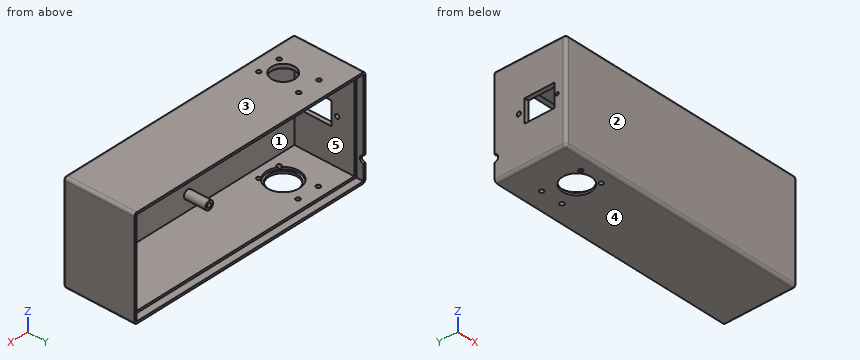
from build123d import *

# Parameters (mm, degrees)
SKETCH1_W           = 176
SKETCH1_H           = 70
BOSS_EXTRUDE1_DEPTH = 50
SKETCH2_W           = 170
SKETCH2_H           = 64
CUT_EXTRUDE1_DEPTH  = 47
SKETCH3_W           = 173
SKETCH3_H           = 67
CUT_EXTRUDE2_DEPTH  = 5
SKETCH4_R           = 3
SKETCH4_R_2         = 1.5
BOSS_EXTRUDE2_DEPTH = 15
CUT_EXTRUDE3_REACH  = 72
SKETCH5_R           = 10
SKETCH5_R_2         = 1.5
SKETCH6_R           = 11.5
CUT_EXTRUDE4_DEPTH  = 1.5
CUT_EXTRUDE5_REACH  = 72
SKETCH7_R           = 8.25
SKETCH7_R_2         = 1.5
SKETCH8_R           = 8.5
CUT_EXTRUDE6_DEPTH  = 1
FILLET1_R           = 2
CUT_EXTRUDE7_REACH  = 178
SKETCH9_R           = 1.5
SKETCH9_R_2         = 1
SKETCH9_W           = 16
SKETCH9_H           = 21
CUT_EXTRUDE8_REACH  = 178
SKETCH10_R          = 2.5


with BuildPart() as part:
    # Sketch1 → Boss-Extrude1 (new body)
    with BuildSketch(Plane(origin=(0, 0, 0), x_dir=(1, 0, 0), z_dir=(0, 1, 0))):
        Rectangle(SKETCH1_W, SKETCH1_H)
    extrude(amount=BOSS_EXTRUDE1_DEPTH)

    # Sketch2 → Cut-Extrude1 (cut)
    with BuildSketch(Plane(origin=(0, 50, 0), x_dir=(1, 0, 0), z_dir=(0, 1, 0))):
        Rectangle(SKETCH2_W, SKETCH2_H)
    extrude(amount=-CUT_EXTRUDE1_DEPTH, mode=Mode.SUBTRACT)

    # Sketch3 → Cut-Extrude2 (cut)
    with BuildSketch(Plane(origin=(0, 50, 0), x_dir=(1, 0, 0), z_dir=(0, 1, 0))):
        Rectangle(SKETCH3_W, SKETCH3_H)
    extrude(amount=-CUT_EXTRUDE2_DEPTH, mode=Mode.SUBTRACT)

    # Sketch4 → Boss-Extrude2 (add)
    with BuildSketch(Plane(origin=(0, 3, 0), x_dir=(1, 0, 0), z_dir=(0, 1, 0))):
        with Locations((-4.8, -27)):
            Circle(SKETCH4_R)
        with Locations((-4.8, -27)):
            Circle(SKETCH4_R_2, mode=Mode.SUBTRACT)
        with Locations((78, -27)):
            Circle(SKETCH4_R)
        with Locations((78, -27)):
            Circle(SKETCH4_R_2, mode=Mode.SUBTRACT)
        with Locations((71.2, 21.5)):
            Circle(SKETCH4_R)
        with Locations((71.2, 21.5)):
            Circle(SKETCH4_R_2, mode=Mode.SUBTRACT)
        with Locations((-3.8, 21.5)):
            Circle(SKETCH4_R)
        with Locations((-3.8, 21.5)):
            Circle(SKETCH4_R_2, mode=Mode.SUBTRACT)
    extrude(amount=BOSS_EXTRUDE2_DEPTH)

    # Sketch5 → Cut-Extrude3 (cut, up to next)
    with BuildSketch(Plane(origin=(0, 0, -35), x_dir=(-1, 0, 0), z_dir=(0, 0, -1)), mode=Mode.PRIVATE) as cut_extrude3_sk1:
        with Locations((58, 20)):
            Circle(SKETCH5_R)
    cut_extrude3_tool1 = extrude(cut_extrude3_sk1.sketch, amount=-CUT_EXTRUDE3_REACH, mode=Mode.PRIVATE) & part.part
    add(cut_extrude3_tool1.solids().sort_by_distance((-58, 20, -35))[0], mode=Mode.SUBTRACT)
    # Sketch5 → Cut-Extrude3 (cut, up to next)
    with BuildSketch(Plane(origin=(0, 0, -35), x_dir=(-1, 0, 0), z_dir=(0, 0, -1)), mode=Mode.PRIVATE) as cut_extrude3_sk2:
        with Locations((65.75, 37.5)):
            Circle(SKETCH5_R_2)
    cut_extrude3_tool2 = extrude(cut_extrude3_sk2.sketch, amount=-CUT_EXTRUDE3_REACH, mode=Mode.PRIVATE) & part.part
    add(cut_extrude3_tool2.solids().sort_by_distance((-65.75, 37.5, -35))[0], mode=Mode.SUBTRACT)
    # Sketch5 → Cut-Extrude3 (cut, up to next)
    with BuildSketch(Plane(origin=(0, 0, -35), x_dir=(-1, 0, 0), z_dir=(0, 0, -1)), mode=Mode.PRIVATE) as cut_extrude3_sk3:
        with Locations((50.25, 37.5)):
            Circle(SKETCH5_R_2)
    cut_extrude3_tool3 = extrude(cut_extrude3_sk3.sketch, amount=-CUT_EXTRUDE3_REACH, mode=Mode.PRIVATE) & part.part
    add(cut_extrude3_tool3.solids().sort_by_distance((-50.25, 37.5, -35))[0], mode=Mode.SUBTRACT)
    # Sketch5 → Cut-Extrude3 (cut, up to next)
    with BuildSketch(Plane(origin=(0, 0, -35), x_dir=(-1, 0, 0), z_dir=(0, 0, -1)), mode=Mode.PRIVATE) as cut_extrude3_sk4:
        with Locations((50.25, 10)):
            Circle(SKETCH5_R_2)
    cut_extrude3_tool4 = extrude(cut_extrude3_sk4.sketch, amount=-CUT_EXTRUDE3_REACH, mode=Mode.PRIVATE) & part.part
    add(cut_extrude3_tool4.solids().sort_by_distance((-50.25, 10, -35))[0], mode=Mode.SUBTRACT)
    # Sketch5 → Cut-Extrude3 (cut, up to next)
    with BuildSketch(Plane(origin=(0, 0, -35), x_dir=(-1, 0, 0), z_dir=(0, 0, -1)), mode=Mode.PRIVATE) as cut_extrude3_sk5:
        with Locations((65.75, 10)):
            Circle(SKETCH5_R_2)
    cut_extrude3_tool5 = extrude(cut_extrude3_sk5.sketch, amount=-CUT_EXTRUDE3_REACH, mode=Mode.PRIVATE) & part.part
    add(cut_extrude3_tool5.solids().sort_by_distance((-65.75, 10, -35))[0], mode=Mode.SUBTRACT)

    # Sketch6 → Cut-Extrude4 (cut)
    with BuildSketch(Plane.XY.offset(-32)):
        with Locations((-58, 20)):
            Circle(SKETCH6_R)
    extrude(amount=-CUT_EXTRUDE4_DEPTH, mode=Mode.SUBTRACT)

    # Sketch7 → Cut-Extrude5 (cut, up to next)
    with BuildSketch(Plane.XY.offset(35), mode=Mode.PRIVATE) as cut_extrude5_sk1:
        with Locations((-58, 20)):
            Circle(SKETCH7_R)
    cut_extrude5_tool1 = extrude(cut_extrude5_sk1.sketch, amount=-CUT_EXTRUDE5_REACH, mode=Mode.PRIVATE) & part.part
    add(cut_extrude5_tool1.solids().sort_by_distance((-58, 20, 35))[0], mode=Mode.SUBTRACT)
    # Sketch7 → Cut-Extrude5 (cut, up to next)
    with BuildSketch(Plane.XY.offset(35), mode=Mode.PRIVATE) as cut_extrude5_sk2:
        with Locations((-65.75, 38)):
            Circle(SKETCH7_R_2)
    cut_extrude5_tool2 = extrude(cut_extrude5_sk2.sketch, amount=-CUT_EXTRUDE5_REACH, mode=Mode.PRIVATE) & part.part
    add(cut_extrude5_tool2.solids().sort_by_distance((-65.75, 38, 35))[0], mode=Mode.SUBTRACT)
    # Sketch7 → Cut-Extrude5 (cut, up to next)
    with BuildSketch(Plane.XY.offset(35), mode=Mode.PRIVATE) as cut_extrude5_sk3:
        with Locations((-50.25, 38)):
            Circle(SKETCH7_R_2)
    cut_extrude5_tool3 = extrude(cut_extrude5_sk3.sketch, amount=-CUT_EXTRUDE5_REACH, mode=Mode.PRIVATE) & part.part
    add(cut_extrude5_tool3.solids().sort_by_distance((-50.25, 38, 35))[0], mode=Mode.SUBTRACT)
    # Sketch7 → Cut-Extrude5 (cut, up to next)
    with BuildSketch(Plane.XY.offset(35), mode=Mode.PRIVATE) as cut_extrude5_sk4:
        with Locations((-65.75, 10)):
            Circle(SKETCH7_R_2)
    cut_extrude5_tool4 = extrude(cut_extrude5_sk4.sketch, amount=-CUT_EXTRUDE5_REACH, mode=Mode.PRIVATE) & part.part
    add(cut_extrude5_tool4.solids().sort_by_distance((-65.75, 10, 35))[0], mode=Mode.SUBTRACT)
    # Sketch7 → Cut-Extrude5 (cut, up to next)
    with BuildSketch(Plane.XY.offset(35), mode=Mode.PRIVATE) as cut_extrude5_sk5:
        with Locations((-50.25, 10)):
            Circle(SKETCH7_R_2)
    cut_extrude5_tool5 = extrude(cut_extrude5_sk5.sketch, amount=-CUT_EXTRUDE5_REACH, mode=Mode.PRIVATE) & part.part
    add(cut_extrude5_tool5.solids().sort_by_distance((-50.25, 10, 35))[0], mode=Mode.SUBTRACT)

    # Sketch8 → Cut-Extrude6 (cut)
    with BuildSketch(Plane(origin=(0, 0, 32), x_dir=(-1, 0, 0), z_dir=(0, 0, -1))):
        with Locations((58, 20)):
            Circle(SKETCH8_R)
    extrude(amount=-CUT_EXTRUDE6_DEPTH, mode=Mode.SUBTRACT)

    # Fillet1
    fillet1_edges = [part.edges().sort_by_distance(p)[0] for p in [
        (0, 0, -35),
        (88, 0, 0),
        (0, 0, 35),
        (-88, 0, 0),
        (-88, 25, -35),
        (88, 25, -35),
        (88, 25, 35),
        (-88, 25, 35),
    ]]
    fillet(fillet1_edges, radius=FILLET1_R)

    # Sketch9 → Cut-Extrude7 (cut, up to next)
    with BuildSketch(Plane.ZY.offset(88), mode=Mode.PRIVATE) as cut_extrude7_sk1:
        with Locations((0, 33)):
            Circle(SKETCH9_R)
    cut_extrude7_tool1 = extrude(cut_extrude7_sk1.sketch, amount=-CUT_EXTRUDE7_REACH, mode=Mode.PRIVATE) & part.part
    add(cut_extrude7_tool1.solids().sort_by_distance((-88, 33, 0))[0], mode=Mode.SUBTRACT)
    # Sketch9 → Cut-Extrude7 (cut, up to next)
    with BuildSketch(Plane.ZY.offset(88), mode=Mode.PRIVATE) as cut_extrude7_sk2:
        with Locations((0, 6)):
            Circle(SKETCH9_R_2)
    cut_extrude7_tool2 = extrude(cut_extrude7_sk2.sketch, amount=-CUT_EXTRUDE7_REACH, mode=Mode.PRIVATE) & part.part
    add(cut_extrude7_tool2.solids().sort_by_distance((-88, 6, 0))[0], mode=Mode.SUBTRACT)
    # Sketch9 → Cut-Extrude7 (cut, up to next)
    with BuildSketch(Plane.ZY.offset(88), mode=Mode.PRIVATE) as cut_extrude7_sk3:
        with Locations((0, 18.5)):
            Rectangle(SKETCH9_W, SKETCH9_H)
    cut_extrude7_tool3 = extrude(cut_extrude7_sk3.sketch, amount=-CUT_EXTRUDE7_REACH, mode=Mode.PRIVATE) & part.part
    add(cut_extrude7_tool3.solids().sort_by_distance((-88, 18.5, 0))[0], mode=Mode.SUBTRACT)

    # Sketch10 → Cut-Extrude8 (cut, up to next)
    with BuildSketch(Plane.ZY.offset(88), mode=Mode.PRIVATE) as cut_extrude8_sk1:
        with Locations((-20, 50)):
            Circle(SKETCH10_R)
    cut_extrude8_tool1 = extrude(cut_extrude8_sk1.sketch, amount=-CUT_EXTRUDE8_REACH, mode=Mode.PRIVATE) & part.part
    add(cut_extrude8_tool1.solids().sort_by_distance((-88, 50, -20))[0], mode=Mode.SUBTRACT)


solid = part.part
Model file for the job. Use its own axes, mm. Face numbers are marked on the shaded views. A direction names the side the tool comes from. Give positions to 0.01 mm unless a question says otherwise; leave off trailing zeros. Loops run counter-clockwise (first coordinate to the right, second up) from the corner with the lowest first, then second, coordinate; pieces in that order, holes last. Notation, with made-up numbers: (31, -1) -> (57, -1) arc R13 cw to (57, 4) -> close; hole circle Ø1 at (-30.5, 58). An arc over 180 degrees is marked (long way). Use a Markdown table: item, result. Add a question column.
(1) Mould opens along Z. For the marked faces 3, 4 and 5 say: +Z half, -Z half, draft (parallel to the pull), parting line (faces both ways), or undercut.
(2) Tool access for the marked faces 1 and 2: list every direction of +Z, -Z, +X, -X, +Y, -Y with a clear straight run to the whole face (end or side of a thin tool).
(3) Slice it at B-B on z = -28.5. List the corners of the cut face in (x, y), and give its area (3 significant figures).
(4) Drop flat-ended pins along their axis: pin 1 Ø6.5 at (x, z) = (-6, 28) entering from +Y; pin 2 Ø16 at (x, y) = (-58, 20) entering from -Z; pin 3 Ø1 at (x, z) = (30, 13.5) entering from +Y; pin 4 Ø3.5 at (y, z) = (33, 0) entering from -X. Give the stop position or say it passes through.
(5) Wall check: line 1 along Z through (x, y) = (78, 12); line 2 along X through (y, z) = (11.25, 27); line 3 along X through (y, z) = (43, 31.5). Give the ranges that are in metal, low to high.
(6) Slice it at A-A on x = -58. Give the number of separate pieces and of enclosed holes in the cut face, and give its area (3 significant figures).
Filled sheet:
| question | item | result |
|---|---|---|
| 1 | face 3 | +Z half |
| 1 | face 4 | -Z half |
| 1 | face 5 | undercut |
| 2 | face 1 | +Y |
| 2 | face 2 | +Z, -Z, +X, -X, -Y |
| 3 | outline | (-88, 2) arc R2 ccw to (-86, 0) -> (86, 0) arc R2 ccw to (88, 2) -> (88, 50) -> (86.5, 50) -> (86.5, 45) -> (85, 45) -> (85, 3) -> (-85, 3) -> (-85, 45) -> (-86.5, 45) -> (-86.5, 50) -> (-88, 50) -> close |
| 3 | area | 793 mm2 |
| 4 | pin 1 | y = 18 |
| 4 | pin 2 | through |
| 4 | pin 3 | y = 3 |
| 4 | pin 4 | x = -88 |
| 5 | line 1 | -35 to -32, 24 to 25.5, 28.5 to 30, 32 to 35 |
| 5 | line 2 | -88 to -85, -7.8 to -6.3, -3.3 to -1.8, 75 to 76.5, 79.5 to 81, 85 to 88 |
| 5 | line 3 | -88 to -85, 85 to 88 |
| 6 | separate pieces | 3 |
| 6 | enclosed holes | 0 |
| 6 | area | 361 mm2 |
